Part model, mm, in its own coordinate system. Give positions to 0.01 mm unless a question says otherwise; leave off trailing zeros. Write each loop counter-clockwise with the first axis right and the second up, starting at its lowest first coordinate (ties: lowest second). Pieces come first, ordered by that corner, then holes.
```python
from build123d import *

# Parameters (mm, degrees)
SKETCH2_W           = 167.005
SKETCH2_H           = 431.8
BOSS_EXTRUDE2_DEPTH = 3.175
SKETCH3_W           = 6.35
SKETCH3_H           = 393.7
CUT_EXTRUDE1_DEPTH  = 232.572450879
SKETCH6_R           = 1.5
CUT_EXTRUDE3_DEPTH  = 232.572450879
SKETCH7_W           = 82.55
SKETCH7_H           = 6.35
CUT_EXTRUDE4_DEPTH  = 232.572450879
SKETCH8_W           = 6.35
SKETCH8_H           = 76.2
BOSS_EXTRUDE3_DEPTH = 6.35


with BuildPart() as part:
    # Sketch2 → Boss-Extrude2 (new, symmetric)
    with BuildSketch(Plane(origin=(0, 0, 0), x_dir=(1, 0, 0), z_dir=(0, 1, 0))):
        Rectangle(SKETCH2_W, SKETCH2_H)
    extrude(amount=BOSS_EXTRUDE2_DEPTH, both=True)

    # Sketch3 → Cut-Extrude1 (cut, through all)
    with BuildSketch(Plane(origin=(0, 3.175, 0), x_dir=(1, 0, 0), z_dir=(0, 1, 0))):
        with Locations((80.3275, 0)):
            Rectangle(SKETCH3_W, SKETCH3_H)
    extrude(amount=-CUT_EXTRUDE1_DEPTH, mode=Mode.SUBTRACT)

    # Sketch6 → Cut-Extrude3 (cut, through all)
    with BuildSketch(Plane(origin=(0, 3.175, 0), x_dir=(1, 0, 0), z_dir=(0, 1, 0))):
        with Locations(Location((19.634985579, -124.677471157, 0), (0, 0, 270))):
            Circle(SKETCH6_R)
        with Locations(Location((19.634985579, -138.1125, 0), (0, 0, 270))):
            Circle(SKETCH6_R)
        with Locations(Location((33.070014421, -124.677471157, 0), (0, 0, 270))):
            Circle(SKETCH6_R)
        with Locations(Location((33.070014421, -138.1125, 0), (0, 0, 270))):
            Circle(SKETCH6_R)
    cut_extrude3 = extrude(amount=-CUT_EXTRUDE3_DEPTH, mode=Mode.SUBTRACT)

    # Mirror1: Cut-Extrude3 across plane
    add(cut_extrude3.mirror(Plane.XY), mode=Mode.SUBTRACT)

    # Sketch7 → Cut-Extrude4 (cut, through all)
    with BuildSketch(Plane(origin=(0, 3.175, 0), x_dir=(1, 0, 0), z_dir=(0, 1, 0))):
        with Locations((42.2275, 200.025)):
            Rectangle(SKETCH7_W, SKETCH7_H)
        with Locations((42.2275, -200.025)):
            Rectangle(SKETCH7_W, SKETCH7_H)
    extrude(amount=-CUT_EXTRUDE4_DEPTH, mode=Mode.SUBTRACT)

    # Sketch8 → Boss-Extrude3 (add)
    with BuildSketch(Plane(origin=(0, 3.175, 0), x_dir=(1, 0, 0), z_dir=(0, 1, 0))):
        with Locations((80.3275, 0)):
            Rectangle(SKETCH8_W, SKETCH8_H)
    extrude(amount=-BOSS_EXTRUDE3_DEPTH)


solid = part.part
```
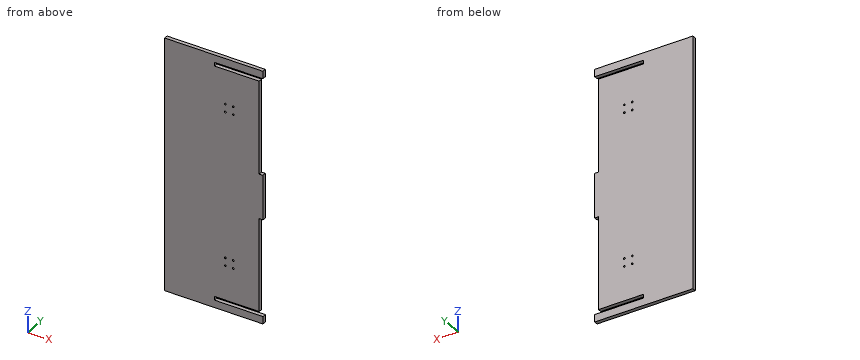
1) Saw through at C-C, the plane z = 155. Write the cut outline in (x, y) (1 decimal).
Answers follow:
outline: (-83.5, -3.2) - (77.2, -3.2) - (77.2, 3.2) - (-83.5, 3.2) - close
2) Pin check, flat tips, straight feed: pin 1 Ø2.5 at (x, z) = (19.63, -138.11) entering from -Y; pin 2 Ø3 at (y, z) = (-1, 118) entering from +X. Stop position of each tip, or through.
Answers follow:
pin 1: passes through
pin 2: stops at x = 77.15
3) Saw through at A-A, the plane x = 41.5. Write the cut outline in (y, z) (3 decimals), then the cut area to 3 significant figures.
Answers follow:
outline: (-3.175, -215.9) - (3.175, -215.9) - (3.175, -203.2) - (-3.175, -203.2) - close; (-3.175, -196.85) - (3.175, -196.85) - (3.175, 196.85) - (-3.175, 196.85) - close; (-3.175, 203.2) - (3.175, 203.2) - (3.175, 215.9) - (-3.175, 215.9) - close
area: 2,660 mm2
4) Saw through at B-B, the plane y = 1.5. Count the separate pieces of the cut face and the enclosed holes in it, then the cut area to 3 significant figures.
Answers follow:
separate pieces: 1
enclosed holes: 8
area: 69,000 mm2
5) Wall check: L1, parallel to Z at x = 29.5, y = -0.75; L2, parallel to X at y = 0.5, z = 185; L3, parallel to X at y = -1, z = 126. Give the ranges that are in metal, low to high.
Answers follow:
L1: z = -215.9 to -203.2, -196.85 to 196.85, 203.2 to 215.9
L2: x = -83.5 to 77.15
L3: x = -83.5 to 18.93, 20.34 to 32.36, 33.78 to 77.15
